Source: CAD feature listing. Evaluate the final solid. Frame: model axes, mm. A direction names the side the tool comes from. Round coordinates to 2 decimals unless told otherwise and drop trailing zeros. Order: outer loops, then holes, each group sorted by start corner. A loop starts at its lowest first (then second) coordinate and runs counter-clockwise, first axis right, second up. Notation, with made-up numbers: (-14, 75) -> (9, 75) arc R9 cw to (9, 91) -> close; hole circle Ø5 at (85.25, -9). An arc over 180 degrees is marked (long way). Write item = value, one per line. Start each with the question number.
(1) Ray query, line 1 (Z direction, x = 7, y = 0); line 2 (Z direction, x = 74.5, y = -0.5); line 3 (X direction, y = 2.5, z = 0.25). Return the intervals inside material, ascending.
(2) Reachability of faces 4 (the face through (220.82, -0.738, -2.345)), 5 (the face through (0, 1, -3)) from +Z, -Z, +X, -X, +Y, -Y: full face, straight path, thin tool, end or side. Return the list, or none.
(3) Contact query for flat-ended pins moving along their axis: pin 1 Ø4.5 at (y, z) = (0, 0) entering from -X; pin 2 Ø1.5 at (x, y) = (158, -1) entering from -Z; pin 3 Ø3 at (x, z) = (152, 3) entering from +Y. Output: stop coordinate, or through.
(4) Cut plane B-B on x = 95. Return the cut outline in (y, z), then the cut area to 3 significant figures.
(5) Draft query along Y for faces 1 (the face through (116.6, -1.08, -4.88)), 2 (the face through (12.222, -0.738, 2.345)), 3 (the face through (230, 1, -3)). Return one class per face: released by +Y, released by -Y, zero draft, split by the parting line, or undercut.
(6) Cut plane A-A on x = 21.5. Return the cut outline in (y, z), then the cut area to 3 significant figures.
Autodesk Inventor part; units mm, degrees
ref_plane "YZ Plane" through (0, 0, 0) normal (1, 0, 0) x (0, 1, 0)
ref_plane "XZ Plane" through (0, 0, 0) normal (0, 1, 0) x (-1, 0, 0)
ref_plane "XY Plane" through (0, 0, 0) normal (0, 0, 1) x (1, 0, 0)
sketch "Sketch_1" plane through (0, 0, 0) normal (0, 0, 1) x (1, 0, 0)
  line L0 (230, 0) -> (0, 0)
  line L1 (0, 0) -> (0, 4.5)
  line L2 (0, 4.5) -> (0.5, 5)
  line L3 (0.5, 5) -> (229.5, 5)
  line L4 (229.5, 5) -> (230, 4.5)
  line L5 (230, 4.5) -> (230, 0)
  line L6 (230, 0) -> (0, 0)
revolve "Revolution1" add sketch "Sketch_1" angle 360 about axis through (230, 0, 0) along (1, 0, 0)
sketch "Sketch2" plane through (0, 0, 0) normal (-1, 0, 0) x (0, 0, 1)
  point P0 (0, 0)
hole "Hole1" at (0, 0, 0) direction (1, 0, 0) diameter 4.917 depth 23.5806 tip angle 120 countersink diameter 6 countersink angle 90
sketch "Sketch3" plane through (230, 0, 0) normal (1, 0, 0) x (0, 0, -1)
  point P0 (0, 0)
hole "Hole2" at (230, 0, 0) direction (-1, 0, 0) diameter 4.917 depth 17.5806 tip angle 120 countersink diameter 6 countersink angle 90
properties part number "SSFRW10-230-MD6-N6_s"
Evaluation:
q1.line_1 = -5 to -2.46, 2.46 to 5
q1.line_2 = -4.97 to 4.97
q1.line_3 = 0.49 to 229.51
q2.face_4 = +X
q2.face_5 = +Z, -Z, -X, +Y, -Y
q3.pin_1 = 23.7
q3.pin_2 = -4.99
q3.pin_3 = 4.77
q4.outline = circle Ø10 at (0, 0)
q4.area = 78.5 mm^2
q5.face_1 = split by the parting line
q5.face_2 = undercut
q5.face_3 = zero draft
q6.outline = circle Ø10 at (0, 0); hole circle Ø4.92 at (0, 0)
q6.area = 59.6 mm^2
